Source: three-view drawing plus pictorial views. Frame: mm from the lowest corner of the part. Coordinates: 2 decimals unless noted, no trailing zeros. Loops run counter-clockwise (first coordinate to the right, second up) from the corner with the lowest first, then second, coordinate; pieces in that order, holes last.
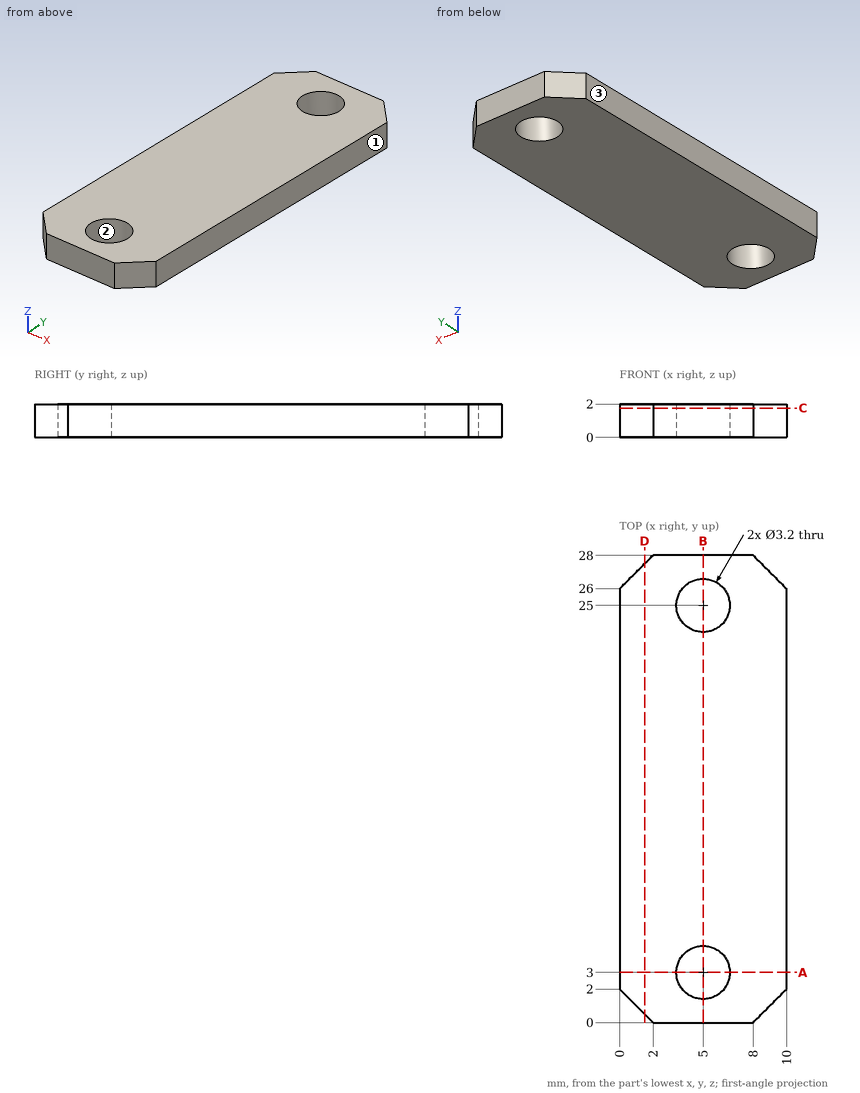
Q1. Section D-D, the plane x = 1.5. Return the cut outline in (y, z), plus the area to 3 significant figures.
Q2. Draft query along X for the marked faces 1, 2 and 3. Return one class per face: +X half, -X half, draft (parallel to the pull), parting line (faces both ways), or undercut.
Q3. Section B-B, the plane x = 5. Return the cut outline in (y, z).
Q4. Section A-A, the plane y = 3. Return the cut outline in (x, z).
Q5. Line query: line 1 along Y through (x, z) = (5, 0.55); line 2 along X through (y, z) = (25, 1.5); line 3 along Y through (x, z) = (4, 0.65). Output: solid intervals per line, ascending.
Q6. Section C-C, the plane z = 1.75. Return the cut outline in (x, y), plus the area to 3 significant figures.
Derived:
1. outline: (0.5, 0) - (27.5, 0) - (27.5, 2) - (0.5, 2) - close
1. area: 54.0 mm2
2. face 1: +X half
2. face 2: undercut
2. face 3: -X half
3. outline: (0, 0) - (1.4, 0) - (1.4, 2) - (0, 2) - close; (4.6, 0) - (23.4, 0) - (23.4, 2) - (4.6, 2) - close; (26.6, 0) - (28, 0) - (28, 2) - (26.6, 2) - close
4. outline: (0, 0) - (3.4, 0) - (3.4, 2) - (0, 2) - close; (6.6, 0) - (10, 0) - (10, 2) - (6.6, 2) - close
5. line 1: y = 0 to 1.4, 4.6 to 23.4, 26.6 to 28
5. line 2: x = 0 to 3.4, 6.6 to 10
5. line 3: y = 0 to 1.75, 4.25 to 23.75, 26.25 to 28
6. outline: (0, 2) - (2, 0) - (8, 0) - (10, 2) - (10, 26) - (8, 28) - (2, 28) - (0, 26) - close; hole circle Ø3.2 at (5, 3); hole circle Ø3.2 at (5, 25)
6. area: 256 mm2
